Design review of the part built by this model. Coordinates are the model's own, in mm. Face numbers are marked on the shaded views. A direction names the side the tool comes from. Coordinates: 2 decimals unless noted, no trailing zeros. Write each loop counter-clockwise with the first axis right and the second up, starting at its lowest first coordinate (ties: lowest second). Pieces come first, ordered by that corner, then holes. Notation, with made-up numbers: (11, -14) - (65, -14) arc R24 ccw to (65, 10) - close; hole circle Ø4 at (62, 38). An arc over 180 degrees is marked (long way). One line per item, written item: value.
from build123d import *

# Parameters (mm, degrees)
F0_W      = 350
F0_H      = 120
F1_DEPTH  = 3
F2_W      = 60
F2_H      = 80
F3_DEPTH  = 3
F4_R      = 5
F5_DEPTH  = 25
F6_W      = 350
F6_H      = 3
F7_DEPTH  = 20
F8_R      = 5
F9_DEPTH  = 25
F11_R     = 2.5
F12_DEPTH = 25


with BuildPart() as f1:
    # F0 (on Top) → F1 (new body)
    with BuildSketch(Plane.XY):
        with Locations((175, -60)):
            Rectangle(F0_W, F0_H)
    extrude(amount=F1_DEPTH)

    # F2 (on face) → F3 (join)
    with BuildSketch(Plane(origin=(0, 0, 0), x_dir=(-1, 0, 0), z_dir=(0, 1, 0))):
        with Locations((30, 40)):
            Rectangle(F2_W, F2_H)
    extrude(amount=-F3_DEPTH)

    # F4 (on face) → F5 (cut)
    with BuildSketch(Plane.XZ.offset(3)):
        with Locations((-30, 40)):
            Circle(F4_R)
    extrude(amount=-F5_DEPTH, mode=Mode.SUBTRACT)

    # F6 (on face) → F7 (join)
    with BuildSketch(Plane.XY.offset(3)):
        with Locations((175, -1.5)):
            Rectangle(F6_W, F6_H)
    extrude(amount=F7_DEPTH)

    # F8 (on face) → F9 (cut)
    with BuildSketch(Plane.XZ.offset(3)):
        with Locations((330, 13)):
            Circle(F8_R)
        with Locations((20, 13)):
            Circle(F8_R)
    extrude(amount=-F9_DEPTH, mode=Mode.SUBTRACT)

    # F11 (on face) → F12 (cut)
    with BuildSketch(Plane.XZ.offset(3)):
        with Locations((175, 13)):
            Circle(F11_R)
    extrude(amount=-F12_DEPTH, mode=Mode.SUBTRACT)


solid = f1.part
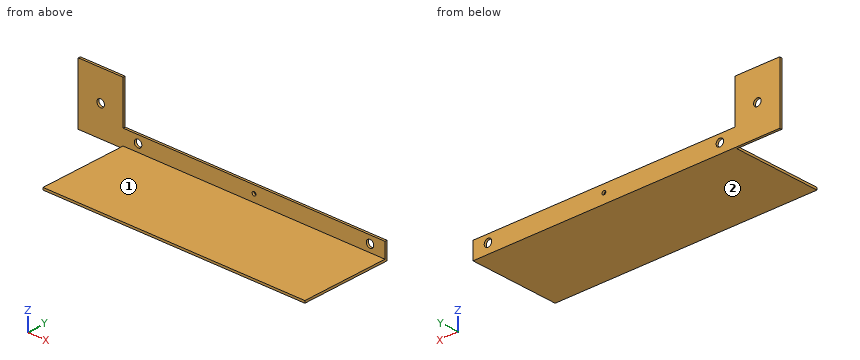
1. Consider section B-B, the plane x = 20. Write out the cut boundary in (y, z).
Answer block:
outline: (-120, 0) - (0, 0) - (0, 8) - (-3, 8) - (-3, 3) - (-120, 3) - close; (-3, 18) - (0, 18) - (0, 23) - (-3, 23) - close
2. Insertion check: pin 1 Ø10 at (x, y) = (211, -63) entering from +Z; pin 2 Ø11.5 at (x, z) = (330, 13) entering from -Y; pin 3 Ø4.5 at (x, z) = (175, 13) entering from -Y; pin 4 Ø1.5 at (x, y) = (127, -1.5) entering from +Z. Each pin has a flat end and moves straight along its axis. Give the tip position at first contact, or say it passes through.
Answer block:
pin 1: stops at z = 3
pin 2: stops at y = -3
pin 3: passes through
pin 4: stops at z = 23
3. For the marked faces 1 and 2, list the 3-axis set-ups (+Z, -Z, +X, -X, +Y, -Y) from which the entire face can be reached by the end or side of a thin tool; tool diameter is ignored.
Answer block:
face 1: +Z, +X, -X, -Y
face 2: -Z, +X, -X, +Y, -Y
4. Consider section C-C, the plane x = 194.5. Write out the cut boundary in (y, z).
Answer block:
outline: (-120, 0) - (0, 0) - (0, 23) - (-3, 23) - (-3, 3) - (-120, 3) - close
5. Consider section A-A, the plane z = 40. Write out the cut boundary in (x, y).
Answer block:
outline: (-60, -3) - (-35, -3) - (-35, 0) - (-60, 0) - close; (-25, -3) - (0, -3) - (0, 0) - (-25, 0) - close
6. Wall thickness on line 1 along Z through (x, y) = (330, -1); line 2 along Y through (x, z) = (-11, 57.5); line 3 along Z through (x, y) = (-30, -1.4): over which ranges is each line inside the solid? List them lowest first.
Answer block:
line 1: z = 0 to 8, 18 to 23
line 2: y = -3 to 0
line 3: z = 0 to 35, 45 to 80
7. Consider section D-D, the plane y = -34. Write out the cut boundary in (x, z).
Answer block:
outline: (0, 0) - (350, 0) - (350, 3) - (0, 3) - close
